from build123d import *

# Parameters (mm, degrees)
F0_W     = 114.3
F0_H     = 114.3
F1_DEPTH = 292.1
F2_T     = -7.62
F3_W     = 41.80703
F3_H     = 120.581752
F4_DEPTH = 70.104


with BuildPart() as f1:
    # F0 (on Top) → F1 (new body)
    with BuildSketch(Plane.XY):
        Rectangle(F0_W, F0_H)
    extrude(amount=F1_DEPTH)

    # F2
    f2_openings = [f1.faces().sort_by_distance(p)[0] for p in [
        (0, 0, 292.1),
    ]]
    offset(amount=F2_T, openings=f2_openings)

    # F3 (on Right) → F4 (cut, symmetric)
    with BuildSketch(Plane.YZ):
        with Locations((0, 233.103248)):
            Rectangle(F3_W, F3_H)
    extrude(amount=F4_DEPTH, both=True, mode=Mode.SUBTRACT)


solid = f1.part
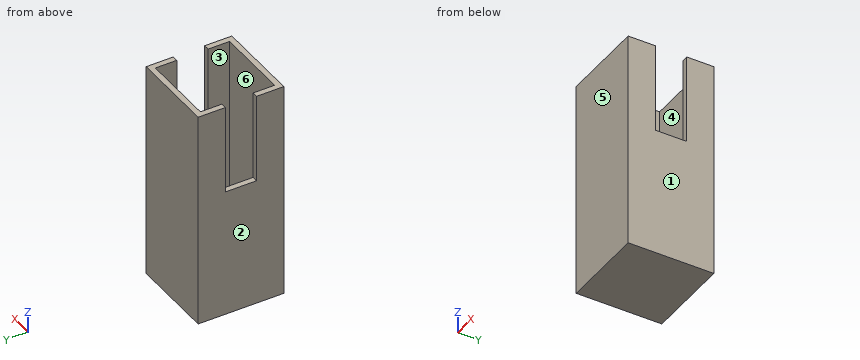
Geometry: final body of the model. Coordinates: model frame, mm. Face numbers are marked on the shaded views. A direction names the side the tool comes from. Round coordinates to 2 decimals unless told otherwise and drop trailing zeros. Write each loop counter-clockwise with the first axis right and the second up, starting at its lowest first coordinate (ties: lowest second). Pieces come first, ordered by that corner, then holes. Notation, with made-up numbers: M -32.75,52 L -25.75,52 A25 cw -25.75,87 Z; hole C -12.75,89.25 d3. An arc over 180 degrees is marked long. Write item = value, one per line.
Item 1: Section query A-A on z = 219. Return loops of the section in (x, y).
Findings:
outline = M -57.15,-57.15 L 57.15,-57.15 L 57.15,-20.9 L 49.53,-20.9 L 49.53,-49.53 L -49.53,-49.53 L -49.53,-20.9 L -57.15,-20.9 Z; M -57.15,20.9 L -49.53,20.9 L -49.53,49.53 L 49.53,49.53 L 49.53,20.9 L 57.15,20.9 L 57.15,57.15 L -57.15,57.15 Z
Item 2: Section query C-C on y = 24.5. Return loops of the section in (x, z), then the cut area to 3 significant figures.
Findings:
outline = M -57.15,0 L 57.15,0 L 57.15,292.1 L 49.53,292.1 L 49.53,7.62 L -49.53,7.62 L -49.53,292.1 L -57.15,292.1 Z
area = 5,210 mm^2
Item 3: Section query B-B on z = 75. Return loops of the section in (x, y), then the cut area to 3 significant figures.
Findings:
outline = M -57.15,-57.15 L 57.15,-57.15 L 57.15,57.15 L -57.15,57.15 Z; hole M -49.53,-49.53 L 49.53,-49.53 L 49.53,49.53 L -49.53,49.53 Z
area = 3,250 mm^2
Item 4: Pull-direction query (X, two-part tool) for the marked faces 1, 2, 3 and 4; classes: pulls with the +X half, pulls with the -X half, needs draft (parallel to the pull), parting line crosses it, or undercut.
Findings:
face_1 = pulls with the +X half
face_2 = pulls with the -X half
face_3 = undercut
face_4 = undercut
Item 5: Access query for the marked faces 5 and 6. Directions: +Z, -Z, +X, -X, +Y, -Y. A direction counts if a zero-diameter tool reaches every point of the face in a straight line with its end or side. Return the directions, or none.
Findings:
face_5 = +Z, -Z, +X, -X, -Y
face_6 = +Z
Item 6: Material intervals for line 1 along X through (y, z) = (-10, 51.5), sorted ascending. Write a range as [from, to].
Findings:
line_1 = [-57.15, -49.53], [49.53, 57.15]
Item 7: Pin query (flat end, axial travel): P1, Ø6, axis at x = -52, y = 0, coming from the +Z side. Return the tip coordinate at first contact, or that it passes through.
Findings:
P1 = 172.81
